from build123d import *

# Parameters (mm, degrees)
SKETCH1_W           = 20
SKETCH1_H           = 20
BOSS_EXTRUDE1_DEPTH = 25


with BuildPart() as part:
    # Sketch1 → Boss-Extrude1 (new body)
    with BuildSketch(Plane.XY):
        with BuildLine():
            Line((-125, 0), (0, 0))
            ThreePointArc((0, 0), (-62.5, -62.5), (-125, 0))
        make_face()
        with Locations((-40, -25)):
            Rectangle(SKETCH1_W, SKETCH1_H, mode=Mode.SUBTRACT)
        with Locations((-85, -25)):
            Rectangle(SKETCH1_W, SKETCH1_H, mode=Mode.SUBTRACT)
    extrude(amount=BOSS_EXTRUDE1_DEPTH)


solid = part.part
Read the model definition and answer for the solid it produces. Units are mm, in the model's axes. A direction names the side the tool comes from. Coordinates: 2 decimals unless noted, no trailing zeros. Order: outer loops, then holes, each group sorted by start corner. A loop starts at its lowest first (then second) coordinate and runs counter-clockwise, first axis right, second up. Notation, with made-up numbers: (13, 79.25) - (50, 79.25) arc R19 ccw to (50, 115.25) - close; hole circle Ø11 at (61, 7). An arc over 180 degrees is marked (long way). Use one line per item in the form item = value.
(1) Section C-C, the plane x = -16.5 is taken. Give the vertices of the cut face in (y, z), then the cut area to 3 significant figures.
Computed values:
outline = (-42.31, 0) - (0, 0) - (0, 25) - (-42.31, 25) - close
area = 1,060 mm²
(2) Section D-D, the plane x = -108 is taken. Give the vertices of the cut face in (y, z), then the cut area to 3 significant figures.
Computed values:
outline = (-42.85, 0) - (0, 0) - (0, 25) - (-42.85, 25) - close
area = 1,070 mm²
(3) For a pull along X with two mould halves and no side action, classify faces 1 (the face through (-75, -25, 12)), 2 (the face through (-63, 0, 12)), 3 (the face through (-61.126, -62.485, 12.325)) as pulls with the +X half, pulls with the -X half, needs draft (parallel to the pull), parting line crosses it, or undercut.
Computed values:
face_1 = undercut
face_2 = needs draft
face_3 = parting line crosses it
(4) Which of the six approach directions +Z, -Z, +X, -X, +Y, -Y give full straight-line access (tool end or side, diameter ignored) to faces 4 (the face through (-50, -25, 12)), 5 (the face through (-62, -24, 0))?
Computed values:
face_4 = +Z, -Z
face_5 = -Z, +X, -X, +Y, -Y
(5) Straight lines are drawn through the part: L1, parallel to X at y = -17.5, z = 10.5; L2, parallel to X at y = -24.5, z = 1; L3, parallel to Y at x = -25, z = 15. For each, find the intervals that lie inside material, in ascending order.
Computed values:
L1 = -122.5 to -95, -75 to -50, -30 to -2.5
L2 = -120 to -95, -75 to -50, -30 to -5
L3 = -50 to 0
(6) Section A-A, the plane x = -45 is taken. Give the vertices of the cut face in (y, z), then the cut area to 3 significant figures.
Computed values:
outline = (-60, 0) - (-35, 0) - (-35, 25) - (-60, 25) - close; (-15, 0) - (0, 0) - (0, 25) - (-15, 25) - close
area = 1,000 mm²
(7) Given pin 1 Ø10 at (x, y) = (-106, -11.5) entering from -Z; pin 2 Ø10 at (y, z) = (-28.5, 16.5) entering from -X; pin 3 Ø6 at (x, z) = (-41, 12) entering from -Y; pin 4 Ø6 at (x, z) = (-81, 17.5) entering from -Y, each flat-ended and moving along its own axis, determine where each tip first touches the part or whether it passes through.
Computed values:
pin_1 = 0
pin_2 = -120.41
pin_3 = -59.7
pin_4 = -60.55
(8) Section B-B, the plane z = 12 is taken. Give the vertices of the cut face in (x, y), then the cut area to 3 significant figures.
Computed values:
outline = (-125, 0) arc R62.5 ccw to (0, 0) - close; hole (-95, -35) - (-75, -35) - (-75, -15) - (-95, -15) - close; hole (-50, -35) - (-30, -35) - (-30, -15) - (-50, -15) - close
area = 5,340 mm²
